Geometry check sheet. Reference: the model listing, model coordinates, mm. A direction names the side the tool comes from. Coordinates: 2 decimals unless noted, no trailing zeros. Order: outer loops, then holes, each group sorted by start corner. A loop starts at its lowest first (then second) coordinate and runs counter-clockwise, first axis right, second up. Notation, with made-up numbers: (50, 5.5) - (100, 5.5) arc R37 cw to (100, 42.5) - close; hole circle Ø2 at (-37, 77). An arc over 180 degrees is marked (long way). Return JSON: item names as keys, results as strings. Group by question number.
Item 1: Draft check along Y on faces 1 (the flat face through (-1, -17, 69.85)), 2 (the flat face through (-1, 1219.2, 51)), 3 (the flat face through (45, 914.4, -1)). Enter one of: pulls with the +Y half, pulls with the -Y half, needs draft (parallel to the pull), parting line crosses it, or undercut.
Item 2: Section check A-A on x = 46.5. Enter the section's corners in (y, z), then the cut area to 3 significant figures.
Item 3: Section check C-C on x = -40.5. Enter the section's corners in (y, z), then the cut area to 3 significant figures.
Item 4: Tool access check on faces 4 (the flat face through (19.05, 958, 1)), 5 (the flat face through (-1, -1219.2, 51)). Record the directions out of +Z, -Z, +X, -X, +Y, -Y that give a thin tool (end or side, any length) a straight path to the whole face; none if there is none.
Item 5: Gauge pin test, flat ends, axial feed: pin 1 (15 mm diameter, centred on x = 48.5, z = -32.5, fed in from +Y); pin 2 (12 mm diameter, centred on x = -25, z = 1.5, fed in from +Y); pin 3 (4 mm diameter, centred on x = 12, z = -41.5, fed in from +Y). Record the tip position at first contact, or that the pin passes through.
Item 6: Scan lines: probe 1 along Y at (x, z) = (54.5, 7); probe 2 along Y at (x, z) = (26, -49); probe 3 along X at (y, z) = (935, 4.5). Record each from-to range of solid material in increasing order.
Item 7: Section check B-B on z = 2.5. Enter the section's corners in (x, y), then the cut area to 3 significant figures.
from build123d import *

# Parameters (mm, degrees)
F0_W     = 139.7
F0_H     = 139.7
F1_DEPTH = 1219.2
F2_SIZE  = 101.6
F3_W     = 88.9
F3_H     = 139.7
F4_DEPTH = 50.8


with BuildPart() as f1:
    # F0 (on Front) → F1 (new body, symmetric)
    with BuildSketch(Plane.XZ):
        Rectangle(F0_W, F0_H)
    extrude(amount=F1_DEPTH, both=True)

    # F2
    f2_edges = [f1.edges().sort_by_distance(p)[0] for p in [
        (0, -1219.2, -69.85),
        (0, 1219.2, -69.85),
    ]]
    chamfer(f2_edges, length=F2_SIZE)

    # F3 (on face) → F4 (cut)
    with BuildSketch(Plane.YZ.offset(69.85)):
        with Locations((958.85, 0)):
            Rectangle(F3_W, F3_H)
    extrude(amount=-F4_DEPTH, mode=Mode.SUBTRACT)


solid = f1.part
Computed:
{
 "1": {"face 1": "needs draft", "face 2": "pulls with the +Y half", "face 3": "undercut"},
 "2": {"outline": "(-1219.2, 31.75) - (-1117.6, -69.85) - (914.4, -69.85) - (914.4, 69.85) - (-1219.2, 69.85) - close; (1003.3, -69.85) - (1117.6, -69.85) - (1219.2, 31.75) - (1219.2, 69.85) - (1003.3, 69.85) - close", "area": "318,000 mm²"},
 "3": {"outline": "(-1219.2, 31.75) - (-1117.6, -69.85) - (1117.6, -69.85) - (1219.2, 31.75) - (1219.2, 69.85) - (-1219.2, 69.85) - close", "area": "330,000 mm²"},
 "4": {"face 4": "+Z, -Z, +X", "face 5": "+Z, -Z, +X, -X, -Y"},
 "5": {"pin 1": "stops at y = 1162.45", "pin 2": "stops at y = 1194.95", "pin 3": "stops at y = 1147.95"},
 "6": {"probe 1": "y = -1194.45 to 914.4, 1003.3 to 1194.45", "probe 2": "y = -1138.45 to 914.4, 1003.3 to 1138.45", "probe 3": "x = -69.85 to 19.05"},
 "7": {"outline": "(-69.85, -1189.95) - (69.85, -1189.95) - (69.85, 914.4) - (19.05, 914.4) - (19.05, 1003.3) - (69.85, 1003.3) - (69.85, 1189.95) - (-69.85, 1189.95) - close", "area": "328,000 mm²"}
}
